Read the model definition and answer for the solid it produces. Units are mm, in the model's axes. A direction names the side the tool comes from. Coordinates: 2 decimals unless noted, no trailing zeros. Loops run counter-clockwise (first coordinate to the right, second up) from the corner with the lowest first, then second, coordinate; pieces in that order, holes last. Notation, with made-up numbers: (-19.5, 4) -> (13.5, 4) arc R25 ccw to (13.5, 33) -> close; hole circle Ø11 at (14, 23.25). An arc over 180 degrees is marked (long way). Answer in a Markdown table with one row per item.
Autodesk Inventor part; units mm, degrees
ref_plane "Work Plane1" through (-24.9, -24.9, 7.7) normal (0, 0, 1) x (1, 0, 0)
ref_plane "Work Plane2" through (-22.9, 24.9, 0.025) normal (0, 1, 0) x (0, 0, 1)
ref_plane "Work Plane3" through (0, 0, 0) normal (0.7071068, -0.7071068, 0) x (0, 0, -1)
sketch "Sketch1" plane through (0, 0, 0) normal (0, 0, 1) x (1, 0, 0)
  circle A0 centre (-10, 20.9) radius 1.875
  circle A1 centre (-10, -20.9) radius 1.875
  circle A2 centre (10, 20.9) radius 1.875
  circle A3 centre (10, -20.9) radius 1.875
  circle A4 centre (20.8, -14.4) radius 2.075
  circle A5 centre (20.8, 14.4) radius 2.075
  circle A6 centre (-20.8, 14.4) radius 2.075
  circle A7 centre (-20.8, -14.4) radius 2.075
  line L0 (16.9, -16.9) -> (-16.9, -16.9)
  line L1 (-16.9, -16.9) -> (-16.9, 16.9)
  line L2 (-16.9, 16.9) -> (16.9, 16.9)
  line L3 (16.9, 16.9) -> (16.9, -16.9)
  line L4 (-17.05, 24.9) -> (-17.05, 22.55)
  line L5 (-17.05, 22.55) -> (-22.55, 17.05)
  line L6 (-22.55, 17.05) -> (-24.9, 17.05)
  line L7 (-24.9, 17.05) -> (-24.9, -17.05)
  line L8 (-24.9, -17.05) -> (-22.55, -17.05)
  line L9 (-22.55, -17.05) -> (-17.05, -22.55)
  line L10 (-17.05, -22.55) -> (-17.05, -24.9)
  line L11 (-17.05, -24.9) -> (17.05, -24.9)
  line L12 (17.05, -24.9) -> (17.05, -22.55)
  line L13 (17.05, -22.55) -> (22.55, -17.05)
  line L14 (22.55, -17.05) -> (24.9, -17.05)
  line L15 (24.9, -17.05) -> (24.9, 17.05)
  line L16 (24.9, 17.05) -> (22.55, 17.05)
  line L17 (22.55, 17.05) -> (17.05, 22.55)
  line L18 (17.05, 22.55) -> (17.05, 24.9)
  line L19 (17.05, 24.9) -> (-17.05, 24.9)
  line L20 (-16.975, 24.825) -> (-16.975, 22.5189)
  line L21 (-16.975, 22.5189) -> (-22.5189, 16.975)
  line L22 (-22.5189, 16.975) -> (-24.825, 16.975)
  line L23 (-24.825, 16.975) -> (-24.825, -16.975)
  line L24 (-24.825, -16.975) -> (-22.5189, -16.975)
  line L25 (-22.5189, -16.975) -> (-16.975, -22.5189)
  line L26 (-16.975, -22.5189) -> (-16.975, -24.825)
  line L27 (-16.975, -24.825) -> (16.975, -24.825)
  line L28 (16.975, -24.825) -> (16.975, -22.5189)
  line L29 (16.975, -22.5189) -> (22.5189, -16.975)
  line L30 (22.5189, -16.975) -> (24.825, -16.975)
  line L31 (24.825, -16.975) -> (24.825, 16.975)
  line L32 (24.825, 16.975) -> (22.5189, 16.975)
  line L33 (22.5189, 16.975) -> (16.975, 22.5189)
  line L34 (16.975, 22.5189) -> (16.975, 24.825)
  line L35 (16.975, 24.825) -> (-16.975, 24.825)
  point P0 (0, 0)
  dimension "d0" = 0.075
ref_plane "Work Plane1" through (-24.9, -24.9, 7.7) normal (0, 0, 1) x (1, 0, 0)
extrude "Extrusion1" add sketch "Sketch1" along normal blind 2.5 from surface at 7.7 contours A0 | A1 | A2 | A3 | A4 | A5 | A6 | A7 | L0 L1 L2 L3 | L35 L34 L33 L32 L31 L30 L29 L28 L27 L26 L25 L24 L23 L22 L21 L20
sketch "Sketch2" plane through (-16.975, -24.825, 10.2) normal (0, 0, 1) x (1, 0, 0)
  line L0 (0, 47.3439) -> (0, 49.65)
  line L1 (-5.5439, 41.8) -> (0, 47.3439)
  line L2 (-7.85, 41.8) -> (-5.5439, 41.8)
  line L3 (-7.85, 7.85) -> (-7.85, 41.8)
  line L4 (-5.5439, 7.85) -> (-7.85, 7.85)
  line L5 (0, 2.3061) -> (-5.5439, 7.85)
  line L6 (0, 0) -> (0, 2.3061)
  line L7 (33.95, 0) -> (0, 0)
  line L8 (33.95, 2.3061) -> (33.95, 0)
  line L9 (39.4939, 7.85) -> (33.95, 2.3061)
  line L10 (41.8, 7.85) -> (39.4939, 7.85)
  line L11 (41.8, 41.8) -> (41.8, 7.85)
  line L12 (39.4939, 41.8) -> (41.8, 41.8)
  line L13 (33.95, 47.3439) -> (39.4939, 41.8)
  line L14 (33.95, 49.65) -> (33.95, 47.3439)
  line L15 (0, 49.65) -> (33.95, 49.65)
  line L16 (33.95, 49.65) -> (41.8, 49.65)
  line L17 (41.8, 49.65) -> (41.8, 41.8)
  line L18 (41.8, 41.8) -> (33.95, 41.8)
  line L19 (33.95, 41.8) -> (33.95, 49.65)
  line L20 (41.8, 49.65) -> (31.8, 49.65)
  line L21 (31.8, 49.65) -> (31.8, 44.65)
  line L22 (36.8, 39.65) -> (41.8, 39.65)
  line L23 (41.8, 39.65) -> (41.8, 49.65)
  line L24 (31.8, 44.65) -> (36.8, 39.65)
  line L25 (36.722, 5.078) -> (-2.772, 44.572)
  line L26 (34.9542, 3.3103) -> (-4.5397, 42.8042)
  line L27 (33.95, 0.7789) -> (-7.0711, 41.8)
  line L28 (27.6579, 0) -> (-7.85, 35.5079)
  point P0 (16.975, 24.825)
  point P1 (31.8, 39.65)
  point P2 (34.9542, 3.3103)
  dimension "d3" = 10
  dimension "d4" = 10
  dimension "d5" = 5
  dimension "d6" = 5
  dimension "d7" = 2.5
  dimension "d8" = 2.5
  dimension "d9" = 5
extrude "Extrusion2" add sketch "Sketch2" along normal blind 31.75 contours L25 L9 L26 L1 | L27 L8 L7 L28 L3 L2
sketch "Sketch3" plane through (10.6829, -24.825, 10.2) normal (-0.7071068, -0.7071068, 0) x (0.7071068, -0.7071068, 0)
  line L0 (0, 0) -> (-50.2157, 0)
  line L1 (0, 0) -> (0, 31.75)
  line L2 (-50.2157, 31.75) -> (0, 31.75)
  line L3 (-50.2157, 0) -> (-50.2157, 31.75)
  line L4 (-50.2157, 15.875) -> (0, 15.875)
  line L5 (-5.7329, 4.625) -> (-44.4829, 4.625)
  line L6 (-44.4829, 4.625) -> (-44.4829, 27.125)
  line L7 (-44.4829, 27.125) -> (-5.7329, 27.125)
  line L8 (-5.7329, 27.125) -> (-5.7329, 4.625)
  line L9 (-5.7329, 4.625) -> (-44.4829, 27.125) construction
  line L10 (-44.4829, 4.625) -> (-5.7329, 27.125) construction
  circle A0 centre (-44.4829, 27.125) radius 1.9375
  circle A1 centre (-44.4829, 15.875) radius 1.9375
  line L11 (-25.1079, 15.875) -> (-5.7329, 15.875)
  circle A2 centre (-15.4204, 15.875) radius 1.9375
  line L12 (-53.0343, 0) -> (2.8186, 0)
  line L13 (-53.0343, 0) -> (-53.0343, 31.75)
  line L14 (2.8186, 31.75) -> (-53.0343, 31.75)
  line L15 (2.8186, 0) -> (2.8186, 31.75)
  line L16 (-0.75, 31) -> (-0.75, 0.75)
  line L17 (-0.75, 0.75) -> (-49.4657, 0.75)
  line L18 (-49.4657, 0.75) -> (-49.4657, 31)
  line L19 (-49.4657, 31) -> (-0.75, 31)
  circle A3 centre (-44.4829, 27.125) radius 2.5375
  circle A4 centre (-44.4829, 15.875) radius 2.5375
  circle A5 centre (-15.4204, 15.875) radius 2.5375
  point P0 (-25.1079, -10.2)
  point P1 (0, 0)
  point P2 (-0.75, 15.875)
  point P3 (-49.4657, 15.875)
  point P4 (0, 0)
  point P5 (0, 31.75)
  dimension "d12" = 38.75
  dimension "d13" = 22.5
  dimension "d14" = 3.875
  dimension "d15" = 3.875
  dimension "d16" = 3.875
  dimension "d21" = 0.75
  dimension "d22" = 5.075
  dimension "d23" = 5.075
  dimension "d24" = 5.075
extrude "Extrusion3" cut sketch "Sketch3" along normal blind 2.5 from surface at -10 contours L0 L3 L4 L18 L17 L16 L1 | L1 L14 L15 L12 | L12 L13 L14 L3 | L4 L16 L19 L18 L3 L2 L1
extrude "Extrusion4" cut sketch "Sketch3" against normal up to surface (5 mm away) contours A1 L6 L4 | L4 L6 A1 | A2 L4 | L4 A2 | L6 A1 L4 | L4 A1 L6 | A0 L6 L7 | L7 L6 A0
extrude "Extrusion5" cut sketch "Sketch3" against normal blind 1.5 from surface at -7.5 contours A4 L6 A1 L4 | L4 A1 L6 A4 | A5 L4 A2 | L4 A2 A5 | A1 L6 L4 | L4 L6 A1 | A4 L4 A1 L6 | L6 A1 L4 A4 | A2 L4 | L4 A2 | A3 L6 A0 L7 | L7 A0 L6 A3 | L6 A1 L4 | L4 A1 L6 | A0 L6 L7 | L7 L6 A0
extrude "Extrusion6" [suppressed]
sketch "Sketch4" plane through (0, 0, 0) normal (0, 1, 0) x (-1, 0, 0)
  line L0 (22.9, 0.025) -> (-22.9, 0.025)
  line L1 (22.9, 42.1) -> (22.9, 0.025)
  line L2 (22.9, 42.1) -> (17.05, 42.1)
  line L3 (17.05, 7.7) -> (17.05, 42.1)
  line L4 (-17.05, 7.7) -> (17.05, 7.7)
  line L5 (-17.05, 7.7) -> (-17.05, 42.1)
  line L6 (-17.05, 42.1) -> (-22.9, 42.1)
  line L7 (-22.9, 0.025) -> (-22.9, 42.1)
  circle A0 centre (19.9, 34.8) radius 2.0625
  circle A1 centre (-19.9, 34.8) radius 2.0625
  circle A2 centre (19.9, 15) radius 2.0625
  circle A3 centre (-19.9, 15) radius 2.0625
  circle A4 centre (10, 3.85) radius 1.5625
  circle A5 centre (-10, 3.85) radius 1.5625
  line L8 (-17.05, 24.9) -> (17.05, 24.9)
  circle A6 centre (0, 24.9) radius 16.25
  point P0 (0, 0)
  dimension "d27" = 32.5
ref_plane "Work Plane2" through (-22.9, 24.9, 0.025) normal (0, 1, 0) x (0, 0, 1)
extrude "Extrusion7" [suppressed]
ref_plane "Work Plane3" through (0, 0, 0) normal (0.7071068, -0.7071068, 0) x (0, 0, -1)
mirror "Mirror1" [suppressed]
extrude "Extrusion8" cut sketch "Sketch2" against normal up to surface (2.5 mm away) contours L0 L15 L21 L24 L19 L18 L22 L11 L10 L9 L25 L1 | L25 L9 L26 L1 | L15 L14 L19 L24 L21 | L26 L9 L8 L27 L2 L1 | L16 L17 L12 L13 L14 | L13 L18 L24 L19 | L24 L18 L19 | L12 L11 L22 L24 L18 | L28 L7 L6 L5 L4 L3
sketch "Sketch5" plane through (-16.975, -24.825, 41.95) normal (0, 0, 1) x (1, 0, 0)
  line L0 (-7.85, 41.8) -> (-7.85, 35.5079)
  line L1 (-7.85, 35.5079) -> (27.6579, 0)
  line L2 (27.6579, 0) -> (33.95, 0)
  line L3 (33.95, 0) -> (33.95, 0.7789)
  line L4 (33.95, 0.7789) -> (-7.0711, 41.8)
  line L5 (-7.0711, 41.8) -> (-7.85, 41.8)
  point P0 (16.975, 24.825)
extrude "Extrusion9" cut sketch "Sketch5" against normal up to surface (34.25 mm away)
fillet "Fillet1" radius 1.25 4 edges at (-18.1075, 16.3397, 41.2) (16.3397, -18.1075, 41.2) (16.3397, -18.1075, 10.95) (-18.1075, 16.3397, 10.95)
properties part number "Mirror Plate Horizontal"
1. A cutting plane is placed at C-C on z = 25.5. Give the vertices of the cut face in (x, y).
A:
| item | result |
|---|---|
| outline | (-18.99, 15.46) -> (-17.22, 13.68) -> (-16.15, 14.74) -> (-12.66, 11.25) -> (-13.72, 10.18) -> (3.33, -6.87) -> (4.4, -5.81) -> (7.89, -9.3) -> (6.83, -10.37) -> (15.46, -18.99) -> (17.22, -17.22) -> (-17.22, 17.22) -> close |
2. A tool of negligible diameter and unlimited length cuts with its end or side. For faces 1 (the flat face through (-14.43, 13.02, 26.11)), 2 (the cylindrical face through (16.062, -17.854, 11.306)), from which of +Z, -Z, +X, -X, +Y, -Y can it reach the whole face along a straight path? Write none if from no direction.
A:
| item | result |
|---|---|
| face 1 | none |
| face 2 | -Z, +X, -Y |
3. Find the intervals of material crossed by probe 1 along X at (y, z) = (-0.5, 39); probe 2 along Y at (x, z) = (-15, 19); probe 3 along Y at (x, z) = (-4.5, 33.5), in increasing order.
A:
| item | result |
|---|---|
| probe 1 | x = -3.04 to 0.5 |
| probe 2 | y = 11.46 to 15 |
| probe 3 | y = 0.96 to 4.5 |
4. A cutting plane is placed at B-B on y = 1. Give the vertices of the cut face in (x, z), and give its area (3 significant figures).
A:
| item | result |
|---|---|
| outline | (-4.54, 10.95) -> (-1, 10.95) -> (-1, 41.2) -> (-4.54, 41.2) -> close |
| area | 107 mm2 |
5. A cutting plane is placed at A-A on z = 17. Give the vertices of the cut face in (x, y), and give its area (3 significant figures).
A:
| item | result |
|---|---|
| outline | (-18.99, 15.46) -> (15.46, -18.99) -> (17.22, -17.22) -> (-17.22, 17.22) -> close |
| area | 122 mm2 |
6. The mould has two halves that part along Y. Classify faces 3 (the flat face through (-1, -1, 41.2)), 4 (the cylindrical face through (-17.854, 16.062, 40.844)), 5 (the flat face through (-14.43, 13.02, 37.36)): pulls with the +Y half, pulls with the -Y half, needs draft (parallel to the pull), parting line crosses it, or undercut.
A:
| item | result |
|---|---|
| face 3 | needs draft |
| face 4 | pulls with the +Y half |
| face 5 | undercut |
7. Given pin 1 Ø10 at (x, z) = (10, 25.5) entering from +Y; pin 2 Ø6 at (y, z) = (6, 24) entering from +X; pin 3 Ø10 at (y, z) = (-14, 28.5) entering from -X, each flat-ended and moving along its own axis, determine where each tip first touches the part or whether it passes through.
A:
| item | result |
|---|---|
| pin 1 | stops at y = -5 |
| pin 2 | stops at x = -3 |
| pin 3 | stops at x = 5.46 |
